The listing builds one solid part. Answer for the finished solid, in the listing's coordinates (mm). A direction names the side the tool comes from. Give positions to 0.01 mm unless a question says otherwise; leave off trailing zeros. Loops run counter-clockwise (first coordinate to the right, second up) from the corner with the lowest first, then second, coordinate; pieces in that order, holes last. Notation, with made-up numbers: M 44.5,9.5 L 65.5,9.5 A19 ccw 65.5,14.5 Z; hole C 81,43.5 d7. An arc over 180 degrees is marked long. Use one line per item in the form item = value. Start each with the question number.
1. Straight lines are drawn through the part: line 1 (X direction, y = 0, z = 4.4); line 2 (Z direction, x = 11, y = 14); line 3 (Y direction, x = 0, z = 3.3). For each, find the intervals that lie inside material, in ascending order. Write a range as from..to.
2. The part is cut by section C-C (z = 2.9). Write down the section's boundary in (x, y).
3. The part is cut by section A-A (y = 0). Write down the section's boundary in (x, z).
4. The part is cut by section D-D (x = 2.5). Write down the section's boundary in (y, z), and give its area (3 significant figures).
5. The mould has two halves that part along X. Classify faces 1 (the face through (20.58, 29.55, 3.58)), 2 (the face through (-0.45, 36.01, 3.58)), 3 (the face through (-27.271, -25.006, 2.564)), 4 (the face through (-0.2, -35.5, 5.2)): released by +X, released by -X, zero draft, split by the parting line, or undercut.
6. For faces 5 (the face through (-1, 1, 0)), 6 (the face through (-8.847, -33.863, 3.578)), determine the directions among +Z, -Z, +X, -X, +Y, -Y from which every point of the face is accessible in a straight line to the end or side of a thin tool.
7. Each of these flat-tipped pins is pushed along its axis until it touches: pin 1 Ø1 at (x, z) = (-10, 2) entering from +Y; pin 2 Ø2 at (x, z) = (-21, 3.5) entering from -Y; pin 3 Ø3 at (x, z) = (6.5, 3) entering from -Y. Where does it stop, or does it pass through?
8. The part is cut by section B-B (x = -7.5). Write down the section's boundary in (y, z), and give its area (3 significant figures).
Autodesk Fusion 360 part; units mm, degrees
sketch "Sketch1" plane through (0, 0, 0) normal (0, 0, 1) x (1, 0, 0)
  circle A0 centre (0, 0) radius 37
  dimension "d1" = 74
extrude "Extrude1" add sketch "Sketch1" along normal blind 3.2
shell "Shell1" thickness 2 removed faces 1 at (-10.1246, 15.5782, 3.2)
sketch "Sketch2" plane through (0, 0, 3.2) normal (0, 0, 1) x (-1, 0, 0)
  circle A0 centre (0, 0) radius 35
  circle A1 centre (0, 0) radius 37
  line L0 (0.7607, -34.9917) -> (-20.2884, -28.5935)
  line L1 (-20.2884, -28.5935) -> (-21.7759, -33.4571)
  line L2 (-21.7759, -33.4571) -> (-0.7372, -39.8892)
  line L3 (-0.7372, -39.8892) -> (0.7607, -34.9917)
  dimension "d5" = 22
extrude "Extrude2" cut sketch "Sketch2" against normal blind 1.2 contours A0 A1 L0 L1 L3 picked at (-0.9203, -35.5996)
extrude "Extrude3" add 1 faces at (35.2522, 4.9796, 3.2) along direction (0, 0, 1) blind 2
Derived:
q1.line_1 = -37..-35, 35..37
q1.line_2 = 0..2
q1.line_3 = -37..-35
q2.outline = M -0.76,34.99 L -0.15,37 A37 ccw long 20.88,30.54 L 20.29,28.59 L 20.11,28.65 A35 cw long Z
q3.outline = M -37,0 L 37,0 L 37,5.2 L 35,5.2 L 35,2 L -35,2 L -35,5.2 L -37,5.2 Z
q4.outline = M -36.92,0 L 36.92,0 L 36.92,2 L -34.91,2 L -34.91,5.2 L -36.92,5.2 Z
q4.area = 154 mm2
q5.face_1 = undercut
q5.face_2 = released by +X
q5.face_3 = split by the parting line
q5.face_4 = zero draft
q6.face_5 = -Z, +X, -X, +Y, -Y
q6.face_6 = +Z
q7.pin_1 = 35.76
q7.pin_2 = -31.13
q7.pin_3 = -36.66
q8.outline = M -36.23,0 L 36.23,0 L 36.23,5.2 L 34.19,5.2 L 34.19,2 L -34.19,2 L -34.19,5.2 L -36.23,5.2 Z
q8.area = 158 mm2
